Check sheet for the modelled part. Datum: model origin and axes. Units: mm. A direction names the side the tool comes from. Round coordinates to 2 decimals unless told otherwise and drop trailing zeros. Write each loop counter-clockwise with the first axis right and the second up, starting at its lowest first coordinate (ties: lowest second). Pieces come first, ordered by that corner, then holes. Notation, with made-up numbers: (61, 31.25) -> (65, 31.25) arc R7 ccw to (65, 40.25) -> close; hole circle Ø5 at (-15.5, 47.25). An arc over 180 degrees is marked (long way). Answer as a JSON object with one key per item and string values. Group by question number.
```python
from build123d import *

# Parameters (mm, degrees)
BOSS_EXTRUDE1_DEPTH      = 1.5875
BOSS_EXTRUDE1_DEPTH_BACK = 1.5875
SKETCH3_R                = 1.5875
SKETCH3_R_2              = 4.7625
CHAMFER1_SIZE            = 1.5875


with BuildPart() as part:
    # Sketch3 → Boss-Extrude1 (new, two sides: drawn at the far end of the back side and taken through both)
    with BuildSketch(Plane.XY.offset(-BOSS_EXTRUDE1_DEPTH_BACK)):
        with BuildLine():
            Line((-12.7, 29.413320739), (-11.957294154, 25.201226576))
            ThreePointArc((-11.957294154, 25.201226576), (-12.067180073, 24.422634348), (-12.614382022, 23.857965597))
            ThreePointArc((-12.614382022, 23.857965597), (0, -26.9875), (12.614382022, 23.857965597))
            ThreePointArc((12.614382022, 23.857965597), (12.067180073, 24.422634348), (11.957294154, 25.201226576))
            Line((11.957294154, 25.201226576), (12.7, 29.413320739))
            Line((12.7, 29.413320739), (12.7, 153.9875))
            Line((12.7, 153.9875), (-12.7, 153.9875))
            Line((-12.7, 153.9875), (-12.7, 29.413320739))
        make_face()
        Circle(SKETCH3_R, mode=Mode.SUBTRACT)
        with Locations((0, 141.2875)):
            Circle(SKETCH3_R_2, mode=Mode.SUBTRACT)
    extrude(amount=BOSS_EXTRUDE1_DEPTH + BOSS_EXTRUDE1_DEPTH_BACK)

    # Chamfer1
    chamfer1_edges = [part.edges().sort_by_distance(p)[0] for p in [
        (-1.5875, 0, 1.5875),
    ]]
    chamfer(chamfer1_edges, length=CHAMFER1_SIZE)


solid = part.part
```
(1) Section check B-B on y = 0. Record the cut outline in (x, z) (1 decimal).
(2) Scan lines: line 1 along Y through (x, z) = (-3.5, -0.95); line 2 along X through (y, z) = (144.5, -0.85); line 3 along X through (y, z) = (-2, 1.2). Record each from-to range of solid material in increasing order.
(3) Section check D-D on y = 132.5. Record the cut outline in (x, z), then the cut area to 3 significant figures.
(4) Go/stop test with flat-tipped pins: pin 1 Ø11 at (x, y) = (0, 141.29) entering from +Z; pin 2 Ø1 at (x, z) = (-17.5, 0.5) entering from -Y; pin 3 Ø3 at (x, y) = (0, 0) entering from +Z; pin 4 Ø1 at (y, z) = (117, -0.5) entering from +X. Record where each tip stops, or that it passes through.
(5) Release check for a two-part mould opening along X. For faces 6 (the flat face through (12.323, 27.278, -0.022)), 7 (the flat face through (0, 153.988, 0)), 8 (the cylindrical face through (-0.34, -1.55, -0.8)), 9 (the cylindrical face through (-1.032, 136.638, -0.022)) record: pulls with the +X half, pulls with the -X half, needs draft (parallel to the pull), parting line crosses it, or undercut.
(6) Access from +Z, -Z, +X, -X, +Y, -Y to the whole of each face (thin tool, end or side, straight path). Record for faces 1 (the flat face through (-12.334, 27.337, -0.022)), 2 (the flat face through (12.7, 91, 0)), 3 (the flat face through (0, 65, -1.588)), 4 (the cylindrical face through (-1, -26.97, -0.02)), 5 (the flat face through (-12.7, 93, 0)).
(7) Section check C-C on z = -1. Record the cut outline in (x, y) (1 decimal), then the cut area to 3 significant figures.
(8) Section check A-A on x = 0. State how many separate pieces and enclosed holes the cut face has, then the cut area to 3 significant figures.
Data:
{
 "1": {"outline": "(-27, -1.6) -> (-1.6, -1.6) -> (-1.6, 0) -> (-3.2, 1.6) -> (-27, 1.6) -> close; (1.6, -1.6) -> (27, -1.6) -> (27, 1.6) -> (3.2, 1.6) -> (1.6, 0) -> close"},
 "2": {"line 1": "y = -26.76 to 138.06, 144.52 to 153.99", "line 2": "x = -12.7 to -3.52, 3.52 to 12.7", "line 3": "x = -26.91 to -1.94, 1.94 to 26.91"},
 "3": {"outline": "(-12.7, -1.59) -> (12.7, -1.59) -> (12.7, 1.59) -> (-12.7, 1.59) -> close", "area": "80.6 mm²"},
 "4": {"pin 1": "stops at z = 1.59", "pin 2": "stops at y = -20.96", "pin 3": "passes through", "pin 4": "stops at x = 12.7"},
 "5": {"face 6": "pulls with the +X half", "face 7": "needs draft", "face 8": "undercut", "face 9": "undercut"},
 "6": {"face 1": "+Z, -Z, -X", "face 2": "+Z, -Z, +X, +Y", "face 3": "-Z, +X, -X, +Y, -Y", "face 4": "+Z, -Z", "face 5": "+Z, -Z, -X, +Y"},
 "7": {"outline": "(-12.7, 29.4) -> (-12, 25.2) arc R1.3 cw to (-12.6, 23.9) arc R27 ccw (long way) to (12.6, 23.9) arc R1.3 cw to (12, 25.2) -> (12.7, 29.4) -> (12.7, 154) -> (-12.7, 154) -> close; hole circle Ø9.5 at (0, 141.3); hole circle Ø3.2 at (0, 0)", "area": "5,460 mm²"},
 "8": {"separate pieces": "3", "enclosed holes": "0", "area": "532 mm²"}
}
